The listing builds one solid part. Answer for the finished solid, in the listing's coordinates (mm). Give positions to 0.01 mm unless a question says otherwise; leave off trailing zeros. Order: outer loops, then holes, each group sorted by start corner. A loop starts at its lowest first (then second) coordinate and runs counter-clockwise, first axis right, second up. Notation, with made-up numbers: (-23.75, 71.5) - (-2.75, 71.5) arc R5 cw to (-2.75, 75.5) - close; hole circle Ø8 at (32, -12). An arc over 180 degrees is marked (long way). Answer in a Markdown table with one row per item.
from build123d import *

# Parameters (mm, degrees)
F0_R     = 1.75
F1_DEPTH = 1.1
F2_R     = 4
F3_R     = 30
F4_R     = 15
F5_R     = 3


with BuildPart() as f1:
    # F0 (on Top) → F1 (new body)
    with BuildSketch(Plane.XY):
        Polygon((-70.716745456, 22.3987678723), (-22.682432743, 0), (-10.682432743, 0), (1.4415796787, 18), (1.4415796787, 30), (-69.2492423021, 30), (-70.4260300789, 26.0807510217), align=None)
        with Locations((-15.682432743, 7)):
            Circle(F0_R, mode=Mode.SUBTRACT)
        with BuildLine():
            Line((-69.3496626194, 24.449523286), (-68.4150438499, 27.5622371752))
            ThreePointArc((-68.4150438499, 27.5622371752), (-66.5470441613, 28.5675118458), (-65.5417694907, 26.6995121572))
            Line((-65.5417694907, 26.6995121572), (-66.4763882602, 23.586798268))
            ThreePointArc((-66.4763882602, 23.586798268), (-68.3443879488, 22.5815235974), (-69.3496626194, 24.449523286))
        make_face(mode=Mode.SUBTRACT)
        with Locations((-8.5584203213, 24.9999999582)):
            Circle(F0_R, mode=Mode.SUBTRACT)
    extrude(amount=F1_DEPTH)

    # F2
    f2_edges = [f1.edges().sort_by_distance(p)[0] for p in [
        (1.44158, 30, 0.55),
    ]]
    fillet(f2_edges, radius=F2_R)

    # F3
    f3_edges = [f1.edges().sort_by_distance(p)[0] for p in [
        (-70.42603, 26.080751, 0.55),
    ]]
    fillet(f3_edges, radius=F3_R)

    # F4
    f4_edges = [f1.edges().sort_by_distance(p)[0] for p in [
        (-22.682433, 0, 0.55),
        (1.44158, 18, 0.55),
        (-10.682433, 0, 0.55),
    ]]
    fillet(f4_edges, radius=F4_R)

    # F5
    f5_edges = [f1.edges().sort_by_distance(p)[0] for p in [
        (-69.249242, 30, 0.55),
        (-70.716745, 22.398768, 0.55),
    ]]
    fillet(f5_edges, radius=F5_R)


solid = f1.part
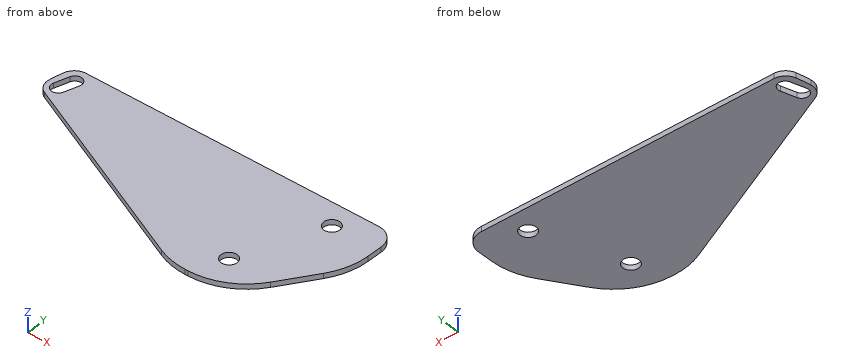
Item 1: Find section A-A on z = 0.3. Count the separate pieces of the cut face and the enclosed holes in it, then the cut area to 3 significant figures.
Answer block:
| item | result |
|---|---|
| separate pieces | 1 |
| enclosed holes | 3 |
| area | 1,460 mm² |
Item 2: Find section C-C on y = 12. Write down the section's boundary in (x, z).
Answer block:
| item | result |
|---|---|
| outline | (-48.42, 0) - (-2.6, 0) - (-2.6, 1.1) - (-48.42, 1.1) - close |
Item 3: Each of these flat-tipped pins is pushed along its axis until it touches: P1, Ø2, axis at x = -7, y = 7.5, coming from the -Z side; P2, Ø2, axis at x = -15.68, y = 7, coming from the -Z side. Where does it stop, or does it pass through?
Answer block:
| item | result |
|---|---|
| P1 | z = 0 |
| P2 | through |
Item 4: Consider line 1 (X direction, y = 25, z = 0.8); line 2 (X direction, y = 26.5, z = 0.75); line 3 (Y direction, x = -18.5, z = 1). Determine where each line is inside the solid, lowest interval first.
Answer block:
| item | result |
|---|---|
| line 1 | -70.44 to -69.18, -66.05 to -10.31, -6.81 to 1.44 |
| line 2 | -70.17 to -68.73, -65.6 to -9.46, -7.66 to 1.41 |
| line 3 | 0 to 30 |
Item 5: Find section B-B on x = -29. Write down the section's boundary in (y, z), then the cut area to 3 significant figures.
Answer block:
| item | result |
|---|---|
| outline | (2.95, 0) - (30, 0) - (30, 1.1) - (2.95, 1.1) - close |
| area | 29.8 mm² |
